from build123d import *

# Parameters (mm, degrees)
SKETCH3_R                = 25.4
BOSS_EXTRUDE1_DEPTH      = 457.2
BOSS_EXTRUDE1_DEPTH_BACK = 457.2
SKETCH4_R                = 9.525
CUT_EXTRUDE2_DEPTH       = 19.05
SKETCH5_R                = 25.4
SKETCH5_R_2              = 23
CUT_EXTRUDE3_DEPTH       = 152.4


with BuildPart() as part:
    # Sketch3 → Boss-Extrude1 (new body, two sides)
    with BuildSketch(Plane.XY) as boss_extrude1_sk:
        Circle(SKETCH3_R)
    extrude(amount=BOSS_EXTRUDE1_DEPTH)
    extrude(boss_extrude1_sk.sketch, amount=-BOSS_EXTRUDE1_DEPTH_BACK)

    # Sketch4 → Cut-Extrude2 (cut)
    with BuildSketch(Plane.XY.offset(-457.2)):
        Circle(SKETCH4_R)
    extrude(amount=CUT_EXTRUDE2_DEPTH, mode=Mode.SUBTRACT)

    # Sketch5 → Cut-Extrude3 (cut)
    with BuildSketch(Plane(origin=(0, 0, -457.2), x_dir=(-1, 0, 0), z_dir=(0, 0, -1))):
        Circle(SKETCH5_R)
        Circle(SKETCH5_R_2, mode=Mode.SUBTRACT)
    extrude(amount=-CUT_EXTRUDE3_DEPTH, mode=Mode.SUBTRACT)


solid = part.part
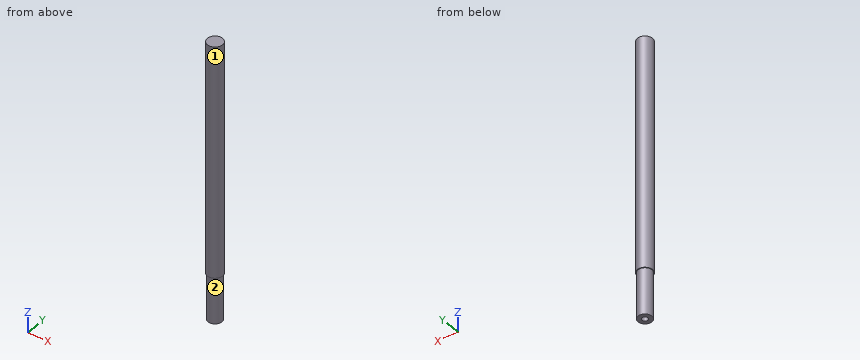
Geometry: final body of the model. Coordinates: model frame, mm. Face numbers are marked on the shaded views. A direction names the side the tool comes from. Give positions to 0.01 mm unless a question says otherwise; leave off trailing zeros. Order: outer loops, then holes, each group sorted by start corner. A loop starts at its lowest first (then second) coordinate and runs counter-clockwise, first axis right, second up. Notation, with made-up numbers: (-10.5, 17.25) -> (6.5, 17.25) arc R11 ccw to (6.5, 31.25) -> close; hole circle Ø9 at (7.25, 3). An arc over 180 degrees is marked (long way). Answer as a JSON object with one key per item and string values.
Q1. Section A-A (y = 0). Output: boundary loops of the cut face in (x, z) (3 decimals).
Entries:
{"outline": "(-25.4, -304.8) -> (-23, -304.8) -> (-23, -457.2) -> (-9.525, -457.2) -> (-9.525, -438.15) -> (9.525, -438.15) -> (9.525, -457.2) -> (23, -457.2) -> (23, -304.8) -> (25.4, -304.8) -> (25.4, 457.2) -> (-25.4, 457.2) -> close"}
Q2. Section C-C (z = -152). Output: boundary loops of the cut face in (x, y).
Entries:
{"outline": "circle Ø50.8 at (0, 0)"}
Q3. Material intervals for probe 1 along Y at (x, z) = (0, -452) (3 decimals); probe 2 along Y at (x, z) = (1, -230), sorted ascending.
Entries:
{"probe 1": "y = -23 to -9.525, 9.525 to 23", "probe 2": "y = -25.38 to 25.38"}
Q4. Access query for the marked faces 1 and 2. Directions: +Z, -Z, +X, -X, +Y, -Y. A direction counts if a zero-diameter tool reaches every point of the face in a straight line with its end or side. Return the directions, or none.
Entries:
{"face 1": "+Z, -Z", "face 2": "-Z"}
Q5. First-contact query: pin 1 (1 mm diameter, centred on x = 8, z = -341.5, fed in from -Y); pin 2 (8 mm diameter, centred on x = -11.5, z = 227.5, fed in from -Y); pin 3 (4 mm diameter, centred on x = -2, z = -39.5, fed in from -Y); pin 4 (21 mm diameter, centred on x = 0, y = 1, fed in from -Z). Flat tips, straight axial feed; report the tip coordinate or a pass-through.
Entries:
{"pin 1": "stops at y = -21.74", "pin 2": "stops at y = -24.27", "pin 3": "stops at y = -25.4", "pin 4": "stops at z = -457.2"}
